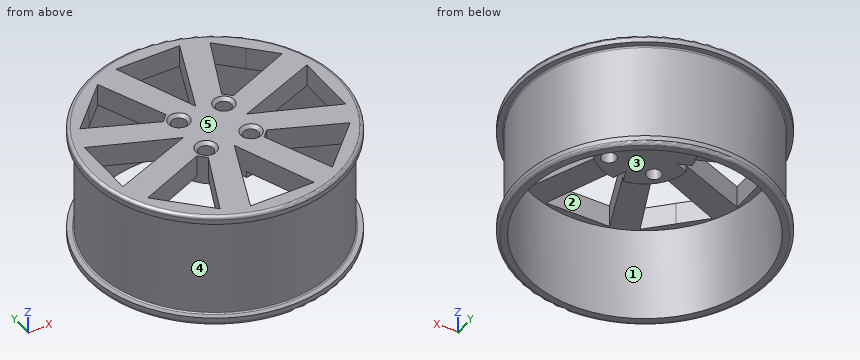
Autodesk Fusion 360 part; units mm, degrees
sketch "Sketch1" plane through (0, 0, 0) normal (0, 1, 0) x (1, 0, 0)
  line L0 (0, 0) -> (190, 0)
  line L1 (0, 0) -> (0, -92.5)
  line L2 (0, -92.5) -> (200, -92.5)
  line L3 (200, -92.5) -> (200, -80)
  line L4 (200, -80) -> (190, -80)
  line L5 (190, -80) -> (190, 0)
  line L6 (190, 80) -> (190, 0)
  line L7 (200, 80) -> (190, 80)
  line L8 (200, 92.5) -> (200, 80)
  line L9 (0, 92.5) -> (200, 92.5)
  line L10 (0, 0) -> (0, 92.5)
  dimension "d3" = 92.5
  dimension "d4" = 200
  dimension "d5" = 12.5
  dimension "d6" = 10
revolve "Revolve1" add sketch "Sketch1" angle 360 about axis through (0, 0, 0) along (0, 0, -1)
sketch "Sketch2" plane through (0, 0, 92.5) normal (0, 0, 1) x (-1, 0, 0)
  circle A0 centre (0, 0) radius 200
  circle A1 centre (35.3553, -35.3553) radius 11.5
  circle A2 centre (35.3553, 35.3553) radius 11.5
  circle A3 centre (-35.3553, 35.3553) radius 11.5
  circle A4 centre (-35.3553, -35.3553) radius 11.5
  dimension "d11" = 23
  dimension "d13" = 360
  dimension "d14" = 100
extrude "Extrude1" cut sketch "Sketch2" against normal through all contours A1 | A2 | A3 | A4
sketch "Sketch3" plane through (0, 0, 92.5) normal (0, 0, 1) x (-1, 0, 0)
  circle A0 centre (35.3553, 35.3553) radius 11.5
  circle A1 centre (-35.3553, 35.3553) radius 11.5
  circle A2 centre (35.3553, -35.3553) radius 11.5
  circle A3 centre (-35.3553, -35.3553) radius 11.5
  circle A4 centre (0, 0) radius 200
  line L0 (0, -175) -> (50, -175)
  line L1 (0, -175) -> (-50, -175)
  line L2 (-50, -175) -> (0, -50)
  line L3 (50, -175) -> (0, -50)
  line L4 (88.3883, -159.099) -> (43.6545, -54.7201)
  line L5 (123.7437, -123.7437) -> (88.3883, -159.099)
  line L6 (123.7437, -123.7437) -> (159.099, -88.3883)
  line L7 (159.099, -88.3883) -> (54.7201, -43.6545)
  line L8 (175, -50) -> (50, 0)
  line L9 (175, 0) -> (175, -50)
  line L10 (175, 0) -> (175, 50)
  line L11 (175, 50) -> (50, 0)
  line L12 (159.099, 88.3883) -> (54.7201, 43.6545)
  line L13 (123.7437, 123.7437) -> (159.099, 88.3883)
  line L14 (123.7437, 123.7437) -> (88.3883, 159.099)
  line L15 (88.3883, 159.099) -> (43.6545, 54.7201)
  line L16 (50, 175) -> (0, 50)
  line L17 (0, 175) -> (50, 175)
  line L18 (0, 175) -> (-50, 175)
  line L19 (-50, 175) -> (0, 50)
  line L20 (-123.7437, 123.7437) -> (-88.3883, 159.099)
  line L21 (-123.7437, 123.7437) -> (-159.099, 88.3883)
  line L22 (-175, 50) -> (-50, 0)
  line L23 (-175, 0) -> (-175, 50)
  line L24 (-175, 0) -> (-175, -50)
  line L25 (-175, -50) -> (-50, 0)
  line L26 (-159.099, -88.3883) -> (-54.7201, -43.6545)
  line L27 (-123.7437, -123.7437) -> (-159.099, -88.3883)
  line L28 (-123.7437, -123.7437) -> (-88.3883, -159.099)
  line L29 (-88.3883, -159.099) -> (-43.6545, -54.7201)
  circle A5 centre (0, 0) radius 70
  line L30 (-88.3883, 159.099) -> (-43.6545, 54.7201)
  line L31 (-159.099, 88.3883) -> (-54.7201, 43.6545)
  dimension "d18" = 50
  dimension "d19" = 125
  dimension "d20" = 50
  dimension "d23" = 140
extrude "Extrude2" cut sketch "Sketch3" against normal through all contours L0 L1 L2 L3 A5 | L2 L3 A5 | L4 L5 L6 L7 A5 | L26 L27 L28 L29 A5 | L8 L9 L10 L11 A5 | L8 L11 A5 | L22 L25 A5 | L22 L23 L24 L25 A5 | L20 L21 A5 L30 L31 | L12 L13 L14 L15 A5 | L16 L19 A5 | L16 L17 L18 L19 A5
sketch "Sketch4" plane through (0, 0, -92.5) normal (0, 0, -1) x (1, 0, 0)
  line L0 (-50, 175) -> (50, 175)
  line L1 (50, 175) -> (0, 50)
  line L2 (0, 50) -> (-50, 175)
  line L3 (50, -175) -> (-50, -175)
  line L4 (-50, -175) -> (0, -50)
  line L5 (0, -50) -> (50, -175)
  line L6 (54.7201, -43.6545) -> (159.099, -88.3883)
  line L7 (159.099, -88.3883) -> (88.3883, -159.099)
  line L8 (88.3883, -159.099) -> (43.6545, -54.7201)
  arc A0 (43.6545, -54.7201) -> (54.7201, -43.6545) centre (0, 0) ccw
  line L9 (-54.7201, 43.6545) -> (-159.099, 88.3883)
  line L10 (-159.099, 88.3883) -> (-88.3883, 159.099)
  line L11 (-88.3883, 159.099) -> (-43.6545, 54.7201)
  arc A1 (-43.6545, 54.7201) -> (-54.7201, 43.6545) centre (0, 0) ccw
  line L12 (43.6545, 54.7201) -> (88.3883, 159.099)
  line L13 (88.3883, 159.099) -> (159.099, 88.3883)
  line L14 (159.099, 88.3883) -> (54.7201, 43.6545)
  arc A2 (54.7201, 43.6545) -> (43.6545, 54.7201) centre (0, 0) ccw
  line L15 (-43.6545, -54.7201) -> (-88.3883, -159.099)
  line L16 (-88.3883, -159.099) -> (-159.099, -88.3883)
  line L17 (-159.099, -88.3883) -> (-54.7201, -43.6545)
  arc A3 (-54.7201, -43.6545) -> (-43.6545, -54.7201) centre (0, 0) ccw
  line L18 (175, 50) -> (175, -50)
  line L19 (175, -50) -> (50, 0)
  line L20 (50, 0) -> (175, 50)
  line L21 (-175, -50) -> (-175, 50)
  line L22 (-175, 50) -> (-50, 0)
  line L23 (-50, 0) -> (-175, -50)
  circle A4 centre (-35.3553, 35.3553) radius 11.5
  circle A5 centre (35.3553, 35.3553) radius 11.5
  circle A6 centre (-35.3553, -35.3553) radius 11.5
  circle A7 centre (35.3553, -35.3553) radius 11.5
  circle A8 centre (0, 0) radius 200
  circle A9 centre (0, 0) radius 70
  circle A10 centre (0, 0) radius 185
  dimension "d25" = 140
  dimension "d26" = 370
extrude "Extrude3" cut sketch "Sketch4" against normal blind 150 contours A10
extrude "Extrude4" cut 1 faces at (-8.9751, 9.1778, -92.5) along direction (0, 0, 1) blind 140
fillet "Fillet1" radius 5 2 edges at (-186.4655, -72.3231, 92.5) (-186.4655, -72.3231, -92.5)
fillet "Fillet2" radius 5 2 edges at (-186.4655, -72.3231, 80) (-186.4655, -72.3231, -80)
chamfer "Chamfer1" distance 5 angle 45 4 edges at (-24.6336, -39.5139, 92.5) (-24.6336, 31.1968, 92.5) (46.0771, 31.1968, 92.5) (46.0771, -39.5139, 92.5)
delete_face "DeleteFace1" 1 faces at (-91.1408, -177.7767, -83.5262)
fillet "Fillet3" radius 2 2 edges at (-177.1422, -68.7069, 80) (-177.1422, -68.7069, -80)
delete_face "DeleteFace2" 1 faces at (-91.1408, -177.7767, 83.5262)
Build history of the part. All positions in model axes, mm. Face numbers are marked on the shaded views. A direction names the side the tool comes from. Give positions to 0.01 mm unless a question says otherwise; leave off trailing zeros. Write each loop counter-clockwise with the first axis right and the second up, starting at its lowest first coordinate (ties: lowest second). Pieces come first, ordered by that corner, then holes. Notation, with made-up numbers: (-35, 11.25) - (1, 11.25) arc R18 ccw to (1, 42.25) - close; hole circle Ø9 at (81, 43.5). An arc over 180 degrees is marked (long way). Use one line per item in the form item = value. Start each with the question number.
1. 3-axis set-ups, long thin cutter, end or side, ignore diameter. For the marked faces 1 and 2: which of +Z, -Z, +X, -X, +Y, -Y reach the whole face in a straight line?
2. Probe line 1 (X direction, y = 81.5, z = 68); line 2 (X direction, y = 0, z = -38); line 3 (Y direction, x = 154, z = 79). List the from-to ranges inside material, lowest first. Write a range as [from, to].
3. Two-plate mould, pull along Y, no slides. Class the marked faces 3, 4 and 5: released by +Y, released by -Y, zero draft, split by the parting line, or undercut.
4. Drop flat-ended pins along their axis: pin 1 Ø1.5 at (y, z) = (30.5, 17) entering from -X; pin 2 Ø10.5 at (x, z) = (-20, 75) entering from -Y; pin 3 Ø2 at (x, z) = (131, -56.5) entering from +Y. Give the stop position or say it passes through.
5. Band-saw the part on B-B on x = -153.5. Count the separate pieces of the cut face and the enclosed holes in it, plus the area to 3 significant figures.
6. Band-saw the part on A-A on z = 5.5. Write the cut outline in (x, y).
Conclusion:
q1.face_1 = -Z
q1.face_2 = +Z, -Z
q2.line_1 = [-171.63, -143.03], [-55.13, -12.6], [12.6, 55.13], [143.03, 171.63]
q2.line_2 = [-190, -185], [185, 190]
q2.line_3 = [-111.74, -93.49], [-86.2, -41.6], [41.6, 86.2], [93.49, 111.74]
q3.face_3 = undercut
q3.face_4 = split by the parting line
q3.face_5 = zero draft
q4.pin_1 = -187.66
q4.pin_2 = -199.15
q4.pin_3 = 138.56
q5.separate_pieces = 4
q5.enclosed_holes = 0
q5.area = 7,780 mm²
q6.outline = circle Ø380 at (0, 0); hole circle Ø370 at (0, 0)
